Geometry check sheet. Reference: the model listing, model coordinates, mm. A direction names the side the tool comes from. Round coordinates to 2 decimals unless told otherwise and drop trailing zeros. Write each loop counter-clockwise with the first axis right and the second up, starting at its lowest first coordinate (ties: lowest second). Pieces come first, ordered by that corner, then holes.
Item 1: Cross-section at C-C (y = 9.5). Enter the section's corners in (x, z), then the cut area to 3 significant figures.
Item 2: Draft check along Z on faces 1 (the face through (13.948, 0.301, -32.115)), 2 (the face through (27.4, 6, -14)), 3 (the face through (26.4, 6, -14)), 4 (the face through (-4.715, 2.521, 4.699)). Enter one of: pulls with the +Z half, pulls with the -Z half, needs draft (parallel to the pull), parting line crosses it, or undercut.
Item 3: Cross-section at A-A (z = -3). Enter the section's corners in (x, y), then the cut area to 3 significant figures.
Item 4: Cross-section at B-B (x = 17.5). Enter the section's corners in (y, z), then the cut area to 3 significant figures.
Item 5: Depth check by flat-ended pin: P1, Ø3.5, axis at y = 4.5, z = -9, coming from the +X side; P2, Ø3.5, axis at y = 7, z = -8.5, coming from the -X side; P3, Ø0.8, axis at y = 5.5, z = -13.5, coming from the +X side; P4, Ø1, axis at y = 8, z = -20.5, coming from the +X side. Enter the tip coordinate at first touch or a pass-through.
Item 6: Scan lines: probe 1 along X at (y, z) = (4, -2); probe 2 along X at (y, z) = (5.75, -24); probe 3 along Z at (x, y) = (20.5, 1.5). Record each from-to range of solid material in increasing order.
Item 7: Access from +Z, -Z, +X, -X, +Y, -Y to the whole of each face (thin tool, end or side, straight path). Record for faces 5 (the face through (14, 6, 0)), 6 (the face through (14, 6, -1)), 7 (the face through (32.099, 0.285, -13.948)).
from build123d import *

# Parameters (mm, degrees)
SKETCH1_W           = 27.4
SKETCH1_H           = 27.4
SKETCH1_W_2         = 25.4
SKETCH1_H_2         = 25.4
BOSS_EXTRUDE1_DEPTH = 35
SKETCH1_3_W         = 37.4
SKETCH1_3_H         = 37.4
SKETCH1_3_W_2       = 27.4
SKETCH1_3_H_2       = 27.4
BOSS_EXTRUDE2_DEPTH = 5
CHAMFER1_SIZE       = 5
CHAMFER1_SIZE_2     = 28.356409098
FILLET1_R           = 1


with BuildPart() as part:
    # Sketch1 → Boss-Extrude1 (new body)
    with BuildSketch(Plane(origin=(0, 0, 0), x_dir=(1, 0, 0), z_dir=(0, 1, 0))):
        with Locations((13.7, 13.7)):
            Rectangle(SKETCH1_W, SKETCH1_H)
        with Locations((13.7, 13.7)):
            Rectangle(SKETCH1_W_2, SKETCH1_H_2, mode=Mode.SUBTRACT)
    extrude(amount=BOSS_EXTRUDE1_DEPTH)

    # Sketch1<3> → Boss-Extrude2 (add)
    with BuildSketch(Plane(origin=(0, 0, 0), x_dir=(1, 0, 0), z_dir=(0, 1, 0))):
        with Locations((13.7, 13.7)):
            Rectangle(SKETCH1_3_W, SKETCH1_3_H)
        with Locations((13.7, 13.7)):
            Rectangle(SKETCH1_3_W_2, SKETCH1_3_H_2, mode=Mode.SUBTRACT)
    extrude(amount=BOSS_EXTRUDE2_DEPTH)

    # Chamfer1
    # the kernel refuses this chamfer: 28.356409098, 5 mm, written as the material it takes off along each edge
    with BuildSketch(Plane(origin=(101.085229169, 35, -27.4), x_dir=(0, 0.2101387607674354, 0.9776715712462578), z_dir=(-1, 0, 0)), Plane(origin=(0, 35, -101.085229169), x_dir=(0.9776715712462578, 0.2101387607674354, 0), z_dir=(0, 0, 1))) as chamfer1_piece_1:
        Polygon((CHAMFER1_SIZE * 0.977671571246, -CHAMFER1_SIZE * 0.210138760767), (-CHAMFER1_SIZE_2 * 0.210138760768, -CHAMFER1_SIZE_2 * 0.977671571249), (0, 0), align=None)
    extrude(amount=174.770458337, mode=Mode.SUBTRACT)
    with BuildSketch(Plane(origin=(27.4, 35, 73.685229169), x_dir=(0.006682531656101585, -0.9999776716360547, 0), z_dir=(0, 0, -1)), Plane(origin=(-73.685229169, 35, 0), x_dir=(0, -0.9999776716360547, 0.006682531656101581), z_dir=(1, 0, 0))) as chamfer1_piece_2:
        Polygon((CHAMFER1_SIZE_2 * 0.999977671639, CHAMFER1_SIZE_2 * 0.00668253165612), (-CHAMFER1_SIZE * 0.0066825316561, CHAMFER1_SIZE * 0.999977671636), (0, 0), align=None)
    extrude(amount=174.770458337, mode=Mode.SUBTRACT)

    # Fillet1
    fillet1_edges = [part.edges().sort_by_distance(p)[0] for p in [
        (-5, 5, -13.7),
        (-5, 2.5, -32.4),
        (13.7, 0, 5),
        (-5, 2.5, 5),
        (32.4, 0, -13.7),
        (32.4, 2.5, 5),
        (13.7, 5, -32.4),
        (32.4, 2.5, -32.4),
        (13.7, 5, 5),
        (32.4, 5, -13.7),
        (-5, 0, -13.7),
        (13.7, 0, -32.4),
    ]]
    fillet(fillet1_edges, radius=FILLET1_R)


solid = part.part
Resolved:
1. outline: (0.5, -26.9) - (26.9, -26.9) - (26.9, -0.5) - (0.5, -0.5) - close; hole (1, -26.4) - (26.4, -26.4) - (26.4, -1) - (1, -1) - close
1. area: 51.4 mm2
2. face 1: pulls with the -Z half
2. face 2: needs draft
2. face 3: undercut
2. face 4: pulls with the +Z half
3. outline: (-5, 1) arc R1 ccw to (-4, 0) - (1, 0) - (1, 12.31) - (0, 6.64) - (0, 5) - (-4, 5) arc R1 ccw to (-5, 4) - close; (26.4, 0) - (31.4, 0) arc R1 ccw to (32.4, 1) - (32.4, 4) arc R1 ccw to (31.4, 5) - (27.4, 5) - (27.4, 6.64) - (26.4, 12.31) - close
3. area: 68.1 mm2
4. outline: (0, -31.4) arc R1 ccw to (1, -32.4) - (4, -32.4) arc R1 ccw to (5, -31.4) - (5, -27.4) - (6.64, -27.4) - (12.31, -26.4) - (0, -26.4) - close; (0, -1) - (12.31, -1) - (6.64, 0) - (5, 0) - (5, 4) arc R1 ccw to (4, 5) - (1, 5) arc R1 ccw to (0, 4) - close
4. area: 68.1 mm2
5. P1: stops at x = 32.4
5. P2: stops at x = 0
5. P3: stops at x = 27.4
5. P4: stops at x = 27.25
6. probe 1: x = -5 to 1, 26.4 to 32.4
6. probe 2: x = 0 to 1, 26.4 to 27.4
6. probe 3: z = -32.4 to -26.4, -1 to 5
7. face 5: +Z, +X, -X, +Y
7. face 6: +Y, -Y
7. face 7: +Z, -Z, +X, -Y
